The model under review builds one solid part; all positions refer to its coordinate system, in mm. Coordinates: 2 decimals unless noted, no trailing zeros. Write each loop counter-clockwise with the first axis right and the second up, starting at its lowest first coordinate (ties: lowest second). Pieces come first, ordered by that corner, then holes.
1) For line 1 (X direction, y = 1.1, z = 139.7); line 2 (X direction, y = 1.7, z = 103); line 3 (X direction, y = 0.65, z = 152.5), list the stretches that pass through material, from the lowest coordinate up.
2) Add section C-C, the plane y = 0.9. State the section outline as (x, z) points.
3) For P1, Ø1, axis at x = 240.5, y = 2.5, coming from the +Z side; P2, Ø8.5, axis at x = 6.35, z = 139.7, coming from the +Y side; P3, Ø1.6, axis at x = 253, y = 1, coming from the +Z side; P4, Ø1, axis at x = 76, y = 1.5, coming from the +Z side, all flat-tipped, find the tip position at first contact; note any pin that passes through.
4) Add section A-A, the plane z = 139.7. State the section outline as (x, y) points (3 decimals).
5) Add section B-B, the plane x = 6.35. State the section outline as (y, z) points (3 decimals), then the cut area to 3 significant figures.
6) Add section D-D, the plane x = 65. State the section outline as (y, z) points (3 decimals), then the cut area to 3 significant figures.
from build123d import *

# Parameters (mm, degrees)
SKETCH1_R           = 4.699
BOSS_EXTRUDE1_DEPTH = 3.175


with BuildPart() as part:
    # Sketch1 → Boss-Extrude1 (new body)
    with BuildSketch(Plane(origin=(0, 0, 0), x_dir=(1, 0, 0), z_dir=(0, 1, 0))):
        Polygon((0, 0), (71.282950754, 0), (304.8, -53.375325558), (304.8, -226.024674442), (71.282950754, -279.4), (0, -279.4), align=None)
        with Locations(Location((6.35, -139.7, 0), (0, 0, 270))):
            Circle(SKETCH1_R, mode=Mode.SUBTRACT)
        Polygon((25.4, -165.1), (177.8, -165.1), (177.8, -177.8), (241.3, -177.8), (241.3, -165.1), (279.4, -165.1), (279.4, -114.3), (241.3, -114.3), (241.3, -101.6), (177.8, -101.6), (177.8, -114.3), (25.4, -114.3), align=None, mode=Mode.SUBTRACT)
    extrude(amount=BOSS_EXTRUDE1_DEPTH)


solid = part.part
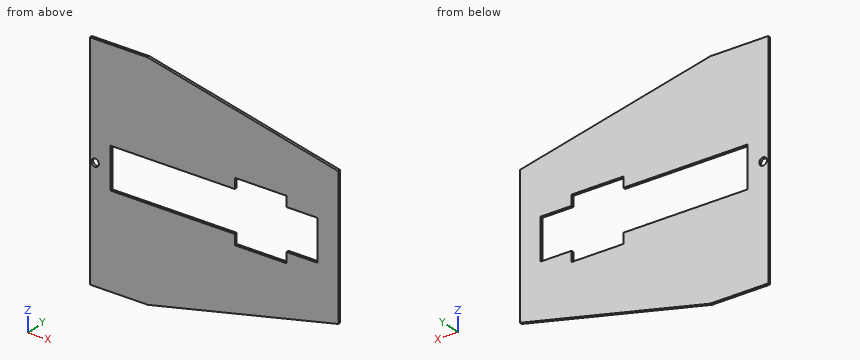
Geometry results:
1. line 1: x = 0 to 1.65, 11.05 to 25.4, 279.4 to 304.8
1. line 2: x = 0 to 177.8, 241.3 to 304.8
1. line 3: x = 0 to 25.4, 279.4 to 304.8
2. outline: (0, 0) - (71.28, 0) - (304.8, 53.38) - (304.8, 226.02) - (71.28, 279.4) - (0, 279.4) - close; hole circle Ø9.4 at (6.35, 139.7); hole (25.4, 114.3) - (177.8, 114.3) - (177.8, 101.6) - (241.3, 101.6) - (241.3, 114.3) - (279.4, 114.3) - (279.4, 165.1) - (241.3, 165.1) - (241.3, 177.8) - (177.8, 177.8) - (177.8, 165.1) - (25.4, 165.1) - close
3. P1: stops at z = 240.84
3. P2: passes through
3. P3: stops at z = 238.05
3. P4: stops at z = 278.44
4. outline: (0, 0) - (1.651, 0) - (1.651, 3.175) - (0, 3.175) - close; (11.049, 0) - (25.4, 0) - (25.4, 3.175) - (11.049, 3.175) - close; (279.4, 0) - (304.8, 0) - (304.8, 3.175) - (279.4, 3.175) - close
5. outline: (0, 0) - (3.175, 0) - (3.175, 135.001) - (0, 135.001) - close; (0, 144.399) - (3.175, 144.399) - (3.175, 279.4) - (0, 279.4) - close
5. area: 857 mm2
6. outline: (0, 0) - (3.175, 0) - (3.175, 114.3) - (0, 114.3) - close; (0, 165.1) - (3.175, 165.1) - (3.175, 279.4) - (0, 279.4) - close
6. area: 726 mm2
